Check sheet for the modelled part. Datum: model origin and axes. Units: mm. A direction names the side the tool comes from. Coordinates: 2 decimals unless noted, no trailing zeros. Write each loop counter-clockwise with the first axis right and the second up, starting at its lowest first coordinate (ties: lowest second). Pieces come first, ordered by that corner, then holes. Notation, with made-up numbers: M 49.25,62 L 105.25,62 A38 ccw 105.25,100 Z; hole C 85,29 d3. An arc over 180 degrees is marked long. Answer as CSV lines item,"result". Start each with the question number.
Q1. Mould release check, pull along X, two halves, no side actions. Record for faces 1 (the flat face through (21, -57.15, 12)), 2 (the cylindrical face through (-24.397, -845.199, -12.69)), 3 (the cylindrical face through (11.654, -14.488, -2.588)): pulls with the +X half, pulls with the -X half, needs draft (parallel to the pull), parting line crosses it, or undercut.
Q2. Sectioned sample at A-A, the plane y = -639.5. Record the cut outline in (x, z) (1 decimal), then the cut area to 3 significant figures.
Q3. Sectioned sample at B-B, the plane y = -133.5. Record the cut outline in (x, z) (1 decimal), then the cut area to 3 significant figures.
Q4. Access from +Z, -Z, +X, -X, +Y, -Y to the whole of each face (thin tool, end or side, straight path). Record for faces 4 (the flat face through (33, -1308.354, 11)), 5 (the cylindrical face through (23.308, -43.063, -5.176)), 6 (the flat face through (-10, -1338.199, -26)).
Q5. Thickness scan on line 1 along X through (y, z) = (-16.75, 0); line 2 along X through (y, z) = (-973.5, 0); line 3 along Y through (x, z) = (-29, -22). Record the ranges inside material, lowest first. Write a range as from..to.
Q6. Depth check by flat-ended pin: pin 1 Ø12 at (x, y) = (8, -755) entering from -Z; pin 2 Ø6 at (x, y) = (-17.5, -508.5) entering from -Z; pin 3 Ø8 at (x, z) = (-38, -2) entering from -Y; pin 4 Ø13 at (x, z) = (0, 0) entering from -Y. Enter the tip coordinate at first touch or a pass-through.
from build123d import *

# Parameters (mm, degrees)
SKETCH2_R          = 4.95
CUT_EXTRUDE1_DEPTH = 25.4
SKETCH5_R          = 27.5
CUT_EXTRUDE3_DEPTH = 1000


with BuildPart() as part:
    # Sketch1 → Revolve1 (revolve)
    with BuildSketch(Plane(origin=(0, 0, 0), x_dir=(0, 0, -1), z_dir=(1, 0, 0))):
        Polygon((0, 0), (-11.938, 0), (-11.938, -28.575), (-23.876, -28.575), (-23.876, -57.15), (-49.2125, -57.15), (-49.2125, -1295.654), (-50.8, -1295.654), (-50.8, -1308.354), (-34.29, -1308.354), (-34.29, -1338.199), (0, -1338.199), align=None)
    revolve(axis=Axis((0, 0, 0), (0, -1, 0)))

    # Sketch2 → Cut-Extrude1 (cut)
    with BuildSketch(Plane(origin=(0, 0, 0), x_dir=(1, 0, 0), z_dir=(0, 1, 0))):
        with Locations(Location((0, 0, 0), (0, 0, 270))):
            Circle(SKETCH2_R)
    extrude(amount=-CUT_EXTRUDE1_DEPTH, mode=Mode.SUBTRACT)

    # Sketch5 → Cut-Extrude3 (cut)
    with BuildSketch(Plane.XZ.offset(1338.199)):
        with Locations(Location((0, 0, 0), (0, 0, 270))):
            Circle(SKETCH5_R)
    extrude(amount=-CUT_EXTRUDE3_DEPTH, mode=Mode.SUBTRACT)


solid = part.part
Output:
1,face 1,"needs draft"
1,face 2,"undercut"
1,face 3,"parting line crosses it"
2,outline,"C 0,0 d98.4; hole C 0,0 d55"
2,area,"5,230 mm^2"
3,outline,"C 0,0 d98.4"
3,area,"7,610 mm^2"
4,face 4,"-Y"
4,face 5,"+Y"
4,face 6,"+Z, -Z, +X, -X, -Y"
5,line 1,"x = -11.94..-4.95, 4.95..11.94"
5,line 2,"x = -49.21..-27.5, 27.5..49.21"
5,line 3,"y = -1308.35..-57.15"
6,pin 1,"stops at z = -49.17"
6,pin 2,"stops at z = -47.03"
6,pin 3,"stops at y = -1338.2"
6,pin 4,"stops at y = -338.2"
